Input: part model. Units: mm. Frame: model coordinates. A direction names the side the tool comes from. Round coordinates to 2 decimals unless told otherwise and drop trailing zeros. Loops run counter-clockwise (first coordinate to the right, second up) from the corner with the lowest first, then second, coordinate; pieces in that order, holes last. Notation, with made-up numbers: M -24,40.5 L 26,40.5 A22 cw 26,70.5 Z; hole C 60,40 d2. An arc over 180 degrees is marked long. Put each result on its own line as item: value. Start each with the question number.
1) Section A-A on x = 149. Output: boundary loops of the cut face in (y, z), plus the area to 3 significant figures.
2) Line query: probe 1 along Y at (x, z) = (173, 0); probe 2 along Y at (x, z) = (165.5, -0.5); probe 3 along Z at (x, y) = (185.5, 0). Output: solid intervals per line, ascending.
3) Draft query along Z for faces 1 (the face through (13.06, 68.335, -15.175)), 2 (the face through (94.17, -10.42, 33.1)), 3 (the face through (226, 0, 49)). Return one class per face: +Z half, -Z half, draft (parallel to the pull), parting line (faces both ways), or undercut.
4) Section C-C on z = 0. Output: boundary loops of the cut face in (x, y).
5) Pin query (flat end, axial travel): pin 1 (11 mm diameter, centred on y = -2.5, z = 3, fed in from +X); pin 2 (12 mm diameter, centred on y = 51.5, z = -4.5, fed in from +X); pin 3 (8 mm diameter, centred on x = 50.5, y = -40, fed in from -Z); pin 4 (8.5 mm diameter, centred on y = 1.5, z = 67.5, fed in from -X). Return the tip coordinate at first contact, or that it passes through.
6) Reachability of faces 4 (the face through (187, 10, 65)), 5 (the face through (162.72, -5.35, -4.1)), 6 (the face through (182, 0, 56.739)) from +Z, -Z, +X, -X, +Y, -Y: full face, straight path, thin tool, end or side. Return the list, or none.
from build123d import *

# Parameters (mm, degrees)
SHELL_1_T                = 3
SKETCH_4_R               = 5.381890803
CUT_EXTRUDE_2_DEPTH      = 10
SWEEP_START              = 143
SWEEP_2_OUTLINE_R        = 6.739132173
SWEEP_2_DEPTH            = 40
SKETCH_7_R               = 5.459251346
CUT_EXTRUDE_3_DEPTH      = 40
EXTRUDE_5_DEPTH          = 80
CUT_EXTRUDE_4_DEPTH      = 10
CUT_EXTRUDE_4_DEPTH_BACK = 90
SKETCH_12_R              = 8.615934325
EXTRUDE_6_DEPTH          = 3


# Read off the part's stored shape, not the designer's step: 扫描2
with BuildPart() as part:
    # 草图1 → 旋转1 (revolve)
    with BuildSketch(Plane(origin=(0, 0, 0), x_dir=(1, 0, 0), z_dir=(0, 1, 0)), mode=Mode.PRIVATE) as revolve_1_sk:
        Polygon((0, 0), (140, 0), (140, 5), (26.491388223, 70), (0, 70), align=None)
    revolve(revolve_1_sk.sketch.rotate(Axis((0, 0, 0), (1, 0, 0)), 180), axis=Axis((0, 0, 0), (1, 0, 0)))

    # 抽壳1
    shell_1_openings = [part.faces().sort_by_distance(p)[0] for p in [
        (0, 0, 0),
    ]]
    offset(amount=SHELL_1_T, openings=shell_1_openings, kind=Kind.INTERSECTION)

    # 草图4 → 切除-拉伸2 (cut)
    with BuildSketch(Plane(origin=(143, 0, 0), x_dir=(0, 0, -1), z_dir=(1, 0, 0))):
        Circle(SKETCH_4_R)
    extrude(amount=-CUT_EXTRUDE_2_DEPTH, mode=Mode.SUBTRACT)

    # 扫描2 outline → 扫描2 (add)
    with BuildSketch(Plane.YZ.offset(SWEEP_START)):
        Circle(SWEEP_2_OUTLINE_R)
    extrude(amount=SWEEP_2_DEPTH)

    # 草图7 → 切除-拉伸3 (cut)
    with BuildSketch(Plane(origin=(143, 0, 0), x_dir=(0, 0, -1), z_dir=(1, 0, 0))):
        Circle(SKETCH_7_R)
    extrude(amount=CUT_EXTRUDE_3_DEPTH, mode=Mode.SUBTRACT)

    # 扫描3: sweep along a curve in space
    with BuildLine() as sweep_3_path:
        ThreePointArc((143, 0, 6.739132173), (143, 4.765286059, 4.765286059), (143, 6.739132173, 0))
        ThreePointArc((143, 6.739132173, 0), (143, 4.765286059, -4.765286059), (143, 0, -6.739132173))
        ThreePointArc((143, 0, -6.739132173), (143, -4.765286059, -4.765286059), (143, -6.739132173, 0))
        ThreePointArc((143, -6.739132173, 0), (143, -4.765286059, 4.765286059), (143, 0, 6.739132173))
    # 草图9 → 扫描3 (sweep)
    with BuildSketch(Plane(origin=(0, 0, 0), x_dir=(1, 0, 0), z_dir=(0, 1, 0))):
        Polygon((143, 6.739132173), (143, 76.739132173), (138, 76.739132173), (138, 9.602351051), align=None)
    sweep(path=sweep_3_path.line)

    # 草图10 → 凸台-拉伸5 (add)
    with BuildSketch(Plane(origin=(143, 0, 0), x_dir=(0, 0, -1), z_dir=(1, 0, 0))):
        with BuildLine():
            Line((-56.739132173, 0), (-56.739132173, 10))
            Line((-56.739132173, 10), (-76.084784331, 10))
            ThreePointArc((-76.084784331, 10), (-76.739132173, 0), (-76.084784331, -10))
            Line((-76.084784331, -10), (-56.739132173, -10))
            Line((-56.739132173, -10), (-56.739132173, 0))
        make_face()
    extrude(amount=EXTRUDE_5_DEPTH)

    # 草图12 → 切除-拉伸4 (cut, two sides: drawn at the far end of the back side and taken through both)
    with BuildSketch(Plane(origin=(223, 0, 0), x_dir=(0, 0, -1), z_dir=(1, 0, 0)).offset(-CUT_EXTRUDE_4_DEPTH_BACK)):
        with Locations((-67.05739748, 0)):
            Circle(SKETCH_12_R)
    extrude(amount=CUT_EXTRUDE_4_DEPTH + CUT_EXTRUDE_4_DEPTH_BACK, mode=Mode.SUBTRACT)

    # 草图11 → 凸台-拉伸6 (add)
    with BuildSketch(Plane(origin=(223, 0, 0), x_dir=(0, 0, -1), z_dir=(1, 0, 0))):
        with BuildLine():
            Line((-76.084784331, 10), (-21.084784331, 10))
            Line((-21.084784331, 10), (-21.084784331, -10))
            Line((-21.084784331, -10), (-76.084784331, -10))
            ThreePointArc((-76.084784331, -10), (-76.739132173, 0), (-76.084784331, 10))
        make_face()
    extrude(amount=EXTRUDE_6_DEPTH)


solid = part.part
Geometry results:
1. outline: M -10,56.74 L 10,56.74 L 10,76.08 A76.74 ccw -10,76.08 Z; C 0,0 d13.48; hole C 0,67.06 d17.23; hole C 0,0 d10.92
1. area: 211 mm²
2. probe 1: y = -6.74 to -5.46, 5.46 to 6.74
2. probe 2: y = -6.72 to -5.44, 5.44 to 6.72
2. probe 3: z = 56.74 to 58.44, 75.67 to 76.74
3. face 1: undercut
3. face 2: parting line
3. face 3: draft
4. outline: M 0,-73 L 27.29,-73 L 138,-9.6 L 138,-76.74 L 143,-76.74 L 143,-6.74 L 183,-6.74 L 183,-5.46 L 143,-5.46 L 143,-5.38 L 139.33,-5.38 L 26.49,-70 L 0,-70 Z; M 0,70 L 26.49,70 L 139.33,5.38 L 143,5.38 L 143,5.46 L 183,5.46 L 183,6.74 L 143,6.74 L 143,76.74 L 138,76.74 L 138,9.6 L 27.29,73 L 0,73 Z
5. pin 1: stops at x = 183
5. pin 2: stops at x = 143
5. pin 3: stops at z = -48.78
5. pin 4: stops at x = 0
6. face 4: +Z, -Z, +X, +Y
6. face 5: +X
6. face 6: +Y, -Y
